Here's the drawing with two shaded views (mm, measured from the low corner). I have some questions. A direction names the side the tool comes from. Round coordinates to 2 decimals unless told otherwise and drop trailing zeros. Loops run counter-clockwise (first coordinate to the right, second up) from the corner with the lowest first, then second, coordinate; pieces in that order, holes last. Notation, with made-up numbers: (77.25, 72) -> (95.25, 72) arc R27 cw to (95.25, 110) -> close; hole circle Ø6 at (-26, -2). An arc over 180 degrees is marked (long way). Write each question's results on one line, items separated by ' | '.
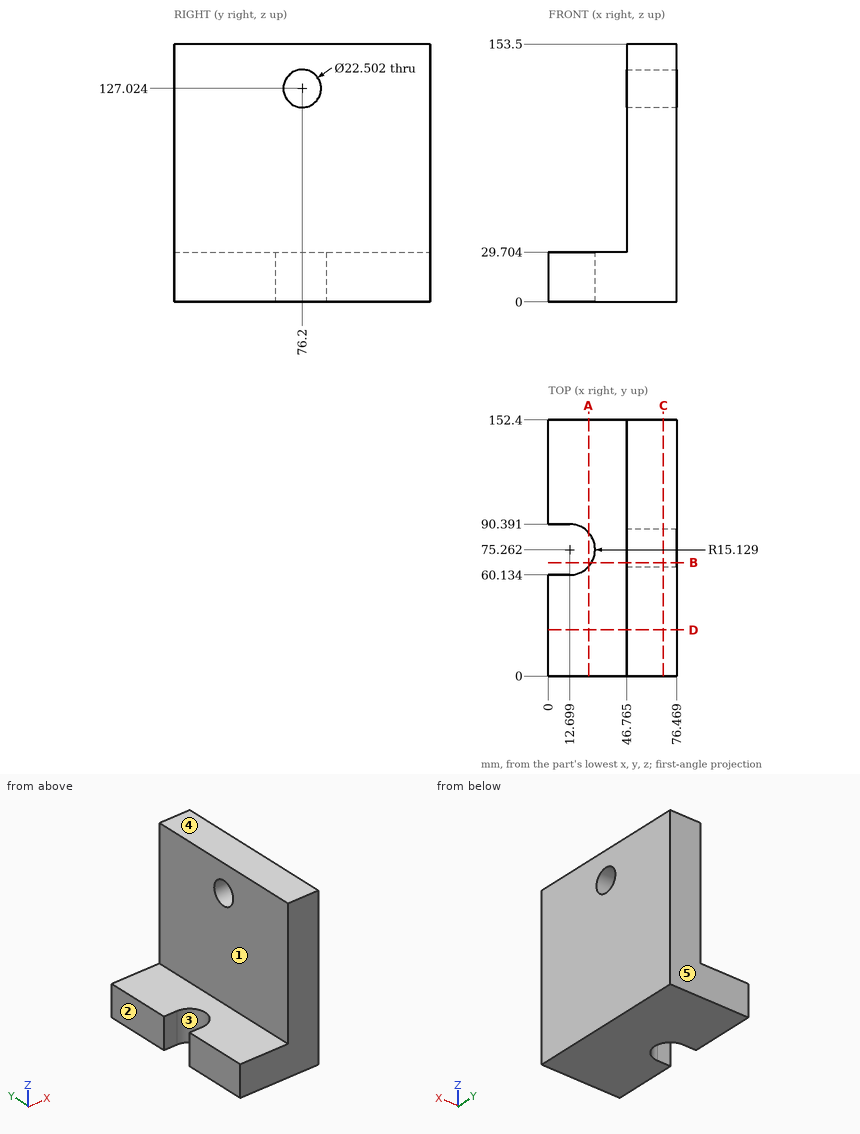
1. If we section it at B-B (y = 67.5): List the corners of the cut face in (x, z) for me (1 decimal), then the cut area to 3 significant figures.
Final values:
outline: (25.7, 0) -> (76.5, 0) -> (76.5, 119.9) -> (46.8, 119.9) -> (46.8, 29.7) -> (25.7, 29.7) -> close; (46.8, 134.2) -> (76.5, 134.2) -> (76.5, 153.5) -> (46.8, 153.5) -> close | area: 4,760 mm2
2. Please list where these lines run through material, in increasing order: line 1 (Z direction, x = 64, y = 76) (1 decimal); line 2 (Z direction, x = 35.5, y = 10); line 3 (X direction, y = 61, z = 81.5) (1 decimal). Write a range as from..to.
Final values:
line 1: 0..115.8, 138.3..153.5 | line 2: 0..29.7 | line 3: 46.8..76.5
3. We'd pull the mould along Y, two halves only. Please class the marked faces 3, 4 and 5: pulls with the +Y half, pulls with the -Y half, needs draft (parallel to the pull), parting line crosses it, or undercut.
Final values:
face 3: undercut | face 4: needs draft | face 5: pulls with the +Y half
4. If we section it at C-C (x = 68.5): List the corners of the cut face in (y, z) for me, then the cut area to 3 significant figures.
Final values:
outline: (0, 0) -> (152.4, 0) -> (152.4, 153.5) -> (0, 153.5) -> close; hole circle Ø22.5 at (76.2, 127.02) | area: 23,000 mm2
5. On a 3-axis mill with a long thin cutter (end or side, diameter ignored), from which of +Z, -Z, +X, -X, +Y, -Y can I reach the whole of each face in a straight line? I mean the marked faces 1 and 2. Say none if no direction works.
Final values:
face 1: +Z, -X, +Y, -Y | face 2: +Z, -Z, -X, +Y, -Y
6. If we section it at A-A (x = 24): List the corners of the cut face in (y, z) for me (1 decimal).
Final values:
outline: (0, 0) -> (65.2, 0) -> (65.2, 29.7) -> (0, 29.7) -> close; (85.3, 0) -> (152.4, 0) -> (152.4, 29.7) -> (85.3, 29.7) -> close
7. If we section it at D-D (y = 27.5): List the corners of the cut face in (x, z) for me (1 decimal).
Final values:
outline: (0, 0) -> (76.5, 0) -> (76.5, 153.5) -> (46.8, 153.5) -> (46.8, 29.7) -> (0, 29.7) -> close
8. Will these pins go through, and if not, where does the flat tip stop? pin 1 (8 mm diameter, centred on y = 23.5, z = 117, fed in from -X) (3 decimals); pin 2 (14 mm diameter, centred on x = 32, y = 86.5, fed in from +Z).
Final values:
pin 1: x = 46.765 | pin 2: z = 29.7
